Part model, mm, in its own coordinate system. Coordinates: 2 decimals unless noted, no trailing zeros. Order: outer loops, then holes, each group sorted by start corner. A loop starts at its lowest first (then second) coordinate and runs counter-clockwise, first axis right, second up.
from build123d import *

# Parameters (mm, degrees)
BOSS_EXTRU_1_DEPTH                                 = 300
ESQUISSE2_W                                        = 0.3
ESQUISSE2_H                                        = 2.4
ENL_V_MAT_EXTRU_1_DEPTH                            = 301.104148588
CHAMBRAGE_POUR_VIS_T_TE_HEXAGONALE_M31_D           = 2.45875
CHAMBRAGE_POUR_VIS_T_TE_HEXAGONALE_M31_CBORE_D     = 6.5
CHAMBRAGE_POUR_VIS_T_TE_HEXAGONALE_M31_CBORE_DEPTH = 3.4
R_P_TITION_LIN_AIRE1_COUNT                         = 15
R_P_TITION_LIN_AIRE1_PITCH                         = 20


with BuildPart() as part:
    # Esquisse1 → Boss.-Extru.1 (new body)
    with BuildSketch(Plane(origin=(0, 0, 0), x_dir=(0, 0, -1), z_dir=(1, 0, 0))):
        Polygon((-4.5, 0), (4.5, 0), (4.5, 3.5), (3.6, 4.4), (3.3, 4.4), (3.3, 5), (3.6, 5), (4.5, 5.9), (4.5, 6.5), (-4.5, 6.5), (-4.5, 5.9), (-3.6, 5), (-3.3, 5), (-3.3, 4.4), (-3.6, 4.4), (-4.5, 3.5), align=None)
    extrude(amount=BOSS_EXTRU_1_DEPTH)

    # Esquisse2 → Enlèv. mat.-Extru.1 (cut, through all)
    with BuildSketch(Plane(origin=(0, 0, 0), x_dir=(0, 0, -1), z_dir=(1, 0, 0))):
        with Locations((4.35, 4.7)):
            Rectangle(ESQUISSE2_W, ESQUISSE2_H)
        with Locations((-4.35, 4.7)):
            Rectangle(ESQUISSE2_W, ESQUISSE2_H)
    extrude(amount=ENL_V_MAT_EXTRU_1_DEPTH, mode=Mode.SUBTRACT)

    # Chambrage pour vis à tête hexagonale M31 (through all)
    with Locations(Plane(origin=(0, 6.5, 0), x_dir=(1, 0, 0), z_dir=(0, 1, 0))):
        with Locations((7.5, 0)):
            chambrage_pour_vis_t_te_hexagonale_m31 = CounterBoreHole(CHAMBRAGE_POUR_VIS_T_TE_HEXAGONALE_M31_D / 2, CHAMBRAGE_POUR_VIS_T_TE_HEXAGONALE_M31_CBORE_D / 2, CHAMBRAGE_POUR_VIS_T_TE_HEXAGONALE_M31_CBORE_DEPTH)

    # Répétition linéaire1: Chambrage pour vis à tête hexagonale M31 ×15
    with Locations(*[(i * R_P_TITION_LIN_AIRE1_PITCH, 0, 0) for i in range(1, R_P_TITION_LIN_AIRE1_COUNT)]):
        add(chambrage_pour_vis_t_te_hexagonale_m31, mode=Mode.SUBTRACT)


solid = part.part
Q1. Mould opens along Z. For faces 1 (the face through (0, 3, 0)), 2 (the face through (289, 3.1, 0)) say: pulls with the +Z half, pulls with the -Z half, needs draft (parallel to the pull), parting line crosses it, or undercut.
Results list:
face 1: needs draft
face 2: undercut
Q2. Pin check, flat tips, straight feed: pin 1 Ø3 at (x, z) = (66.5, 0) entering from +Y; pin 2 Ø1.5 at (x, y) = (126, 4.5) entering from +Z. Stop position of each tip, or through.
Results list:
pin 1: stops at y = 3.1
pin 2: stops at z = 4.2
Q3. Wall check: line 1 along Z through (x, y) = (148, 3.75); line 2 along Y through (x, z) = (84, -3.5); line 3 along Z through (x, y) = (107.5, 1.25). Give the ranges that are in metal, low to high.
Results list:
line 1: z = -4.2 to -3.21, 3.21 to 4.2
line 2: y = 0 to 4.4, 5 to 6.5
line 3: z = -4.5 to -1.23, 1.23 to 4.5
Q4. Cut at A-A on y = 1.5. Count the separate pieces of the cut face and the enclosed holes in it, and give its area (3 significant figures).
Results list:
separate pieces: 1
enclosed holes: 15
area: 2,630 mm2
Q5. Cut at B-B on x = 55. Write the cut outline in (y, z).
Results list:
outline: (0, -4.5) - (3.5, -4.5) - (3.5, -4.2) - (3.8, -4.2) - (4.4, -3.6) - (4.4, -3.3) - (5, -3.3) - (5, -3.6) - (5.6, -4.2) - (5.9, -4.2) - (5.9, -4.5) - (6.5, -4.5) - (6.5, 4.5) - (5.9, 4.5) - (5.9, 4.2) - (5.6, 4.2) - (5, 3.6) - (5, 3.3) - (4.4, 3.3) - (4.4, 3.6) - (3.8, 4.2) - (3.5, 4.2) - (3.5, 4.5) - (0, 4.5) - close
